Here's how the part is built. I have some questions about the finished solid (model axes, mm). Face numbers are marked on the shaded views. Give positions to 0.01 mm unless a question says otherwise; leave off trailing zeros. Loops run counter-clockwise (first coordinate to the right, second up) from the corner with the lowest first, then second, coordinate; pieces in that order, holes last.
Q1. I need wall thicknesses on probe 1 along Z at (x, y) = (-4.5, 0.5); probe 2 along Z at (x, y) = (5, -5); probe 3 along Y at (x, z) = (1.5, -11.5). Which ranges of each line are inside material? Lowest first, please.
Q2. I'm going to push flat-ended pins straight in: P1, Ø8, axis at x = -2.5, y = -5, coming from the -Z side; P2, Ø5, axis at x = 1.5, z = -6.5, coming from the +Y side; P3, Ø3, axis at x = 4.5, z = 12.5, coming from the +Y side; P4, Ø6, axis at y = -6, z = 2, coming from the +X side. Where does each tip first touch, or does it pass through?
Q3. Thinking about a two-plate mould opening in Z: for the marked faces 1, 2 and 3, which applies, pulls with the +Z half, pulls with the -Z half, needs draft (parallel to the pull), parting line crosses it, or undercut?
Q4. Suppose I cut it at C-C (z = -11). List the corners of the cut face in (x, y) for me, and give its area (3 significant figures).
Q5. Suppose I cut it at A-A (y = 0). List the corners of the cut face in (x, z) for me.
```python
from build123d import *

# Parameters (mm, degrees)
CHAMFER1_SIZE = 0.3


with BuildPart() as part:
    # Sketch1 → Revolve1 (revolve)
    with BuildSketch(Plane(origin=(0, 0, 0), x_dir=(1, 0, 0), z_dir=(0, 1, 0))):
        Polygon((0, -17.618415179), (-7.5, -17.618415179), (-7.5, -16.118415179), (-5, -16.118415179), (-5, 13.881584821), (-4.4, 13.881584821), (-4.4, 15.081584821), (-5, 15.081584821), (-5, 16.381584821), (0, 16.381584821), align=None)
    revolve(axis=Axis((0, 0, -34.457254464), (0, 0, 1)))

    # Chamfer1
    chamfer1_edges = [part.edges().sort_by_distance(p)[0] for p in [
        (5, 0, -16.381584821),
        (7.5, 0, 16.118415179),
        (7.5, 0, 17.618415179),
    ]]
    chamfer(chamfer1_edges, length=CHAMFER1_SIZE)


solid = part.part
```
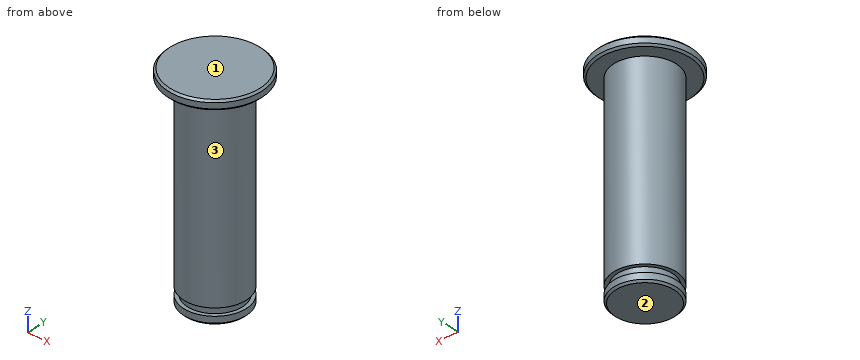
Solutions:
1. probe 1: z = -16.38 to -15.08, -13.88 to 17.62
1. probe 2: z = 16.12 to 17.62
1. probe 3: y = -4.77 to 4.77
2. P1: stops at z = -16.38
2. P2: stops at y = 5
2. P3: stops at y = 4
2. P4: stops at x = 4
3. face 1: pulls with the +Z half
3. face 2: pulls with the -Z half
3. face 3: needs draft
4. outline: circle Ø10 at (0, 0)
4. area: 78.5 mm2
5. outline: (-7.5, 16.42) - (-7.2, 16.12) - (-5, 16.12) - (-5, -13.88) - (-4.4, -13.88) - (-4.4, -15.08) - (-5, -15.08) - (-5, -16.08) - (-4.7, -16.38) - (4.7, -16.38) - (5, -16.08) - (5, -15.08) - (4.4, -15.08) - (4.4, -13.88) - (5, -13.88) - (5, 16.12) - (7.2, 16.12) - (7.5, 16.42) - (7.5, 17.32) - (7.2, 17.62) - (-7.2, 17.62) - (-7.5, 17.32) - close
